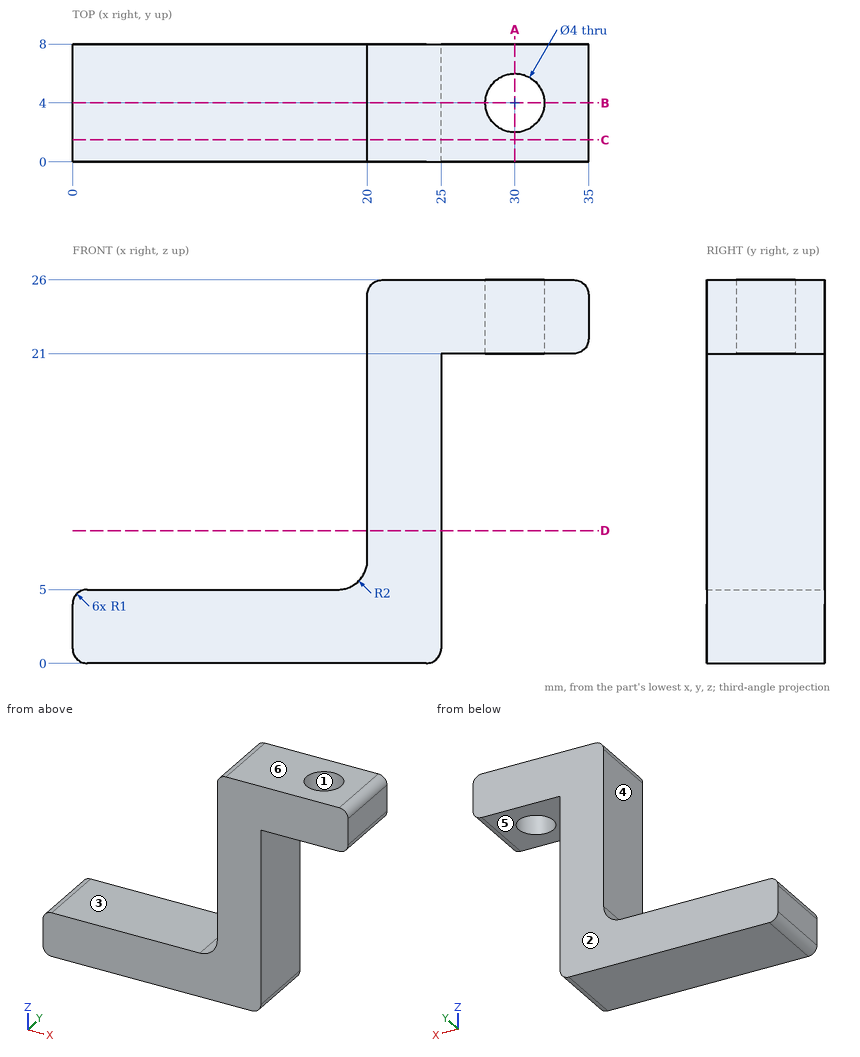
Here's the drawing with two shaded views (mm, measured from the low corner). I have some questions. A direction names the side the tool comes from. Round coordinates to 2 decimals unless told otherwise and drop trailing zeros. Order: outer loops, then holes, each group sorted by start corner. A loop starts at its lowest first (then second) coordinate and runs counter-clockwise, first axis right, second up. Notation, with made-up numbers: (-10, -29) -> (45, -29) arc R26 ccw to (45, 9) -> close; hole circle Ø2 at (4, -11.75). An arc over 180 degrees is marked (long way). Use a Markdown table: item, result. Add a question column.
(1) For pin 1 Ø2.5 at (y, z) = (5.5, 11.5) entering from +X; pin 2 Ø4 at (x, y) = (27.5, 5) entering from -Z; pin 3 Ø2.5 at (x, y) = (30, 4) entering from +Z; pin 4 Ø12 at (x, z) = (23.5, 20) entering from -Y, each with a flat end and sliding along its axis, tell me the tip position at first contact or that it passes through.
(2) I need wall thicknesses on line 1 along Y through (x, z) = (30, 22.05); line 2 along Z through (x, y) = (13, 0.75); line 3 along X through (y, z) = (5.5, 9.25). Which ranges of each line are inside material? Lowest first, please.
(3) If we mould it in two halves opening along Y, with no side actions, what happens to the marked faces 1, 2 and 3? For each: released by +Y, released by -Y, zero draft, split by the parting line, or undercut.
(4) Suppose I cut it at A-A, the plane x = 30. Please give me the cut outline in (y, z), and give its area (3 significant figures).
(5) Suppose I cut it at B-B, the plane y = 4. Please give me the cut outline in (x, z).
(6) For the marked faces 4, 5 and 6, which set-ups out of +Z, -Z, +X, -X, +Y, -Y let a thin tool reach every point of the face, with its end or its side?
(7) Suppose I cut it at D-D, the plane z = 9. Please give me the cut outline in (x, y).
(8) Suppose I cut it at C-C, the plane y = 1.5. Please give me the cut outline in (x, z).
Verdict:
| question | item | result |
|---|---|---|
| 1 | pin 1 | x = 25 |
| 1 | pin 2 | z = 21 |
| 1 | pin 3 | through |
| 1 | pin 4 | y = 0 |
| 2 | line 1 | 0 to 2, 6 to 8 |
| 2 | line 2 | 0 to 5 |
| 2 | line 3 | 20 to 25 |
| 3 | face 1 | undercut |
| 3 | face 2 | released by +Y |
| 3 | face 3 | zero draft |
| 4 | outline | (0, 21) -> (2, 21) -> (2, 26) -> (0, 26) -> close; (6, 21) -> (8, 21) -> (8, 26) -> (6, 26) -> close |
| 4 | area | 20.0 mm2 |
| 5 | outline | (0, 1) arc R1 ccw to (1, 0) -> (24, 0) arc R1 ccw to (25, 1) -> (25, 21) -> (28, 21) -> (28, 26) -> (21, 26) arc R1 ccw to (20, 25) -> (20, 7) arc R2 cw to (18, 5) -> (1, 5) arc R1 ccw to (0, 4) -> close; (32, 21) -> (34, 21) arc R1 ccw to (35, 22) -> (35, 25) arc R1 ccw to (34, 26) -> (32, 26) -> close |
| 6 | face 4 | +Z, -X, +Y, -Y |
| 6 | face 5 | -Z, +X, +Y, -Y |
| 6 | face 6 | +Z, +X, -X, +Y, -Y |
| 7 | outline | (20, 0) -> (25, 0) -> (25, 8) -> (20, 8) -> close |
| 8 | outline | (0, 1) arc R1 ccw to (1, 0) -> (24, 0) arc R1 ccw to (25, 1) -> (25, 21) -> (34, 21) arc R1 ccw to (35, 22) -> (35, 25) arc R1 ccw to (34, 26) -> (21, 26) arc R1 ccw to (20, 25) -> (20, 7) arc R2 cw to (18, 5) -> (1, 5) arc R1 ccw to (0, 4) -> close |
